Check sheet for the modelled part. Datum: model origin and axes. Units: mm. Round coordinates to 2 decimals unless told otherwise and drop trailing zeros. Write each loop counter-clockwise with the first axis right and the second up, starting at its lowest first coordinate (ties: lowest second). Pieces come first, ordered by that corner, then holes. Notation, with made-up numbers: (81.5, 49) -> (118.5, 49) arc R12 cw to (118.5, 58) -> close; hole circle Ø8 at (49.25, -6.75). An arc over 180 degrees is marked (long way). One line per item, written item: value.
from build123d import *

# Parameters (mm, degrees)
SKETCH_1_R          = 25
EXTRUDE_1_DEPTH     = 6
SKETCH_2_R          = 1.5
CUT_EXTRUDE_1_DEPTH = 10


with BuildPart() as part:
    # 草图1 → 凸台-拉伸1 (new body)
    with BuildSketch(Plane(origin=(0, 0, 0), x_dir=(1, 0, 0), z_dir=(0, 1, 0))):
        with Locations(Location((0, 0, 0), (0, 0, 270))):
            Circle(SKETCH_1_R)
    extrude(amount=EXTRUDE_1_DEPTH)

    # 草图2 → 切除-拉伸1 (cut)
    with BuildSketch(Plane(origin=(0, 6, 0), x_dir=(1, 0, 0), z_dir=(0, 1, 0))):
        with Locations(Location((9.75, 0, 0), (0, 0, 270))):
            Circle(SKETCH_2_R)
        with Locations(Location((0, -9.75, 0), (0, 0, 270))):
            Circle(SKETCH_2_R)
        with Locations(Location((-9.75, 0, 0), (0, 0, 270))):
            Circle(SKETCH_2_R)
        with Locations(Location((0, 9.75, 0), (0, 0, 270))):
            Circle(SKETCH_2_R)
        with Locations(Location((0, 0, 0), (0, 0, 270))):
            Circle(SKETCH_2_R)
        with Locations(Location((-20, 0, 0), (0, 0, 270))):
            Circle(SKETCH_2_R)
        with Locations(Location((-10, 17.320508076, 0), (0, 0, 270))):
            Circle(SKETCH_2_R)
        with Locations(Location((10, 17.320508076, 0), (0, 0, 270))):
            Circle(SKETCH_2_R)
        with Locations(Location((20, 0, 0), (0, 0, 270))):
            Circle(SKETCH_2_R)
        with Locations(Location((10, -17.320508076, 0), (0, 0, 270))):
            Circle(SKETCH_2_R)
        with Locations(Location((-10, -17.320508076, 0), (0, 0, 270))):
            Circle(SKETCH_2_R)
    extrude(amount=-CUT_EXTRUDE_1_DEPTH, mode=Mode.SUBTRACT)


solid = part.part
Item 1: Material ranges on line 1 along X through (y, z) = (2.55, 0); line 2 along X through (y, z) = (3.85, 16.5); line 3 along X through (y, z) = (1.5, -9.75), recorded low to high.
Result set:
line 1: -25 to -21.5, -18.5 to -11.25, -8.25 to -1.5, 1.5 to 8.25, 11.25 to 18.5, 21.5 to 25
line 2: -18.78 to -11.26, -8.74 to 8.74, 11.26 to 18.78
line 3: -23.02 to -1.5, 1.5 to 23.02
Item 2: Sectioned sample at D-D (y = 2.9). State how many separate pieces and enclosed holes the cut face has, then the cut area to 3 significant figures.
Result set:
separate pieces: 1
enclosed holes: 11
area: 1,890 mm^2
Item 3: Sectioned sample at A-A (z = 0). Enter the section's corners in (x, y).
Result set:
outline: (-25, 0) -> (-21.5, 0) -> (-21.5, 6) -> (-25, 6) -> close; (-18.5, 0) -> (-11.25, 0) -> (-11.25, 6) -> (-18.5, 6) -> close; (-8.25, 0) -> (-1.5, 0) -> (-1.5, 6) -> (-8.25, 6) -> close; (1.5, 0) -> (8.25, 0) -> (8.25, 6) -> (1.5, 6) -> close; (11.25, 0) -> (18.5, 0) -> (18.5, 6) -> (11.25, 6) -> close; (21.5, 0) -> (25, 0) -> (25, 6) -> (21.5, 6) -> close
Item 4: Release check for a two-part mould opening along X. For faces 1 (the cylindrical face through (-18.735, 3.042, 0.806)), 2 (the cylindrical face through (7.509, 2.958, 23.846)), 3 (the flat face through (0, 0, 5)) record: pulls with the +X half, pulls with the -X half, needs draft (parallel to the pull), parting line crosses it, or undercut.
Result set:
face 1: undercut
face 2: parting line crosses it
face 3: needs draft
Item 5: Sectioned sample at C-C (x = 20). Enter the section's corners in (y, z), then the cut area to 3 significant figures.
Result set:
outline: (0, -15) -> (6, -15) -> (6, -1.5) -> (0, -1.5) -> close; (0, 1.5) -> (6, 1.5) -> (6, 15) -> (0, 15) -> close
area: 162 mm^2
Item 6: Sectioned sample at B-B (x = 0). Enter the section's corners in (y, z).
Result set:
outline: (0, -25) -> (6, -25) -> (6, -11.25) -> (0, -11.25) -> close; (0, -8.25) -> (6, -8.25) -> (6, -1.5) -> (0, -1.5) -> close; (0, 1.5) -> (6, 1.5) -> (6, 8.25) -> (0, 8.25) -> close; (0, 11.25) -> (6, 11.25) -> (6, 25) -> (0, 25) -> close
Item 7: Depth check by flat-ended pin: pin 1 (3.5 mm diameter, centred on x = -20, z = 0, fed in from +Y); pin 2 (1.8 mm diameter, centred on x = 0, z = -9.75, fed in from +Y); pin 3 (2 mm diameter, centred on y = 5.5, z = 14, fed in from -X); pin 4 (2 mm diameter, centred on y = 3, z = -19.5, fed in from +X). Enter the tip coordinate at first touch or a pass-through.
Result set:
pin 1: y = 6
pin 2: through
pin 3: x = -21.35
pin 4: x = 16.82
